```python
from build123d import *

# Parameters (mm, degrees)
SKETCH1_W           = 25.4
SKETCH1_H           = 25.4
BOSS_EXTRUDE1_DEPTH = 19.05
BOSS_EXTRUDE2_DEPTH = 25.4


with BuildPart() as part:
    # Sketch1 → Boss-Extrude1 (new body)
    with BuildSketch(Plane(origin=(0, 0, 0), x_dir=(1, 0, 0), z_dir=(0, 1, 0))):
        with Locations((12.7, 12.7)):
            Rectangle(SKETCH1_W, SKETCH1_H)
    extrude(amount=BOSS_EXTRUDE1_DEPTH)

    # Sketch3 → Boss-Extrude2 (add)
    with BuildSketch(Plane(origin=(0, 19.05, 0), x_dir=(1, 0, 0), z_dir=(0, 1, 0))):
        with BuildLine():
            Line((0, 0), (0, 9.1694))
            ThreePointArc((0, 9.1694), (6.483744919, 6.483744919), (9.1694, 0))
            Line((9.1694, 0), (0, 0))
        make_face()
    extrude(amount=BOSS_EXTRUDE2_DEPTH)


solid = part.part
```
Check sheet for the modelled part. Datum: model origin and axes. Units: mm. A direction names the side the tool comes from. Round coordinates to 2 decimals unless told otherwise and drop trailing zeros. Order: outer loops, then holes, each group sorted by start corner. A loop starts at its lowest first (then second) coordinate and runs counter-clockwise, first axis right, second up.
1) Section check D-D (x = 19.75). Record the boundary of the cut face in (y, z), and give its area (3 significant figures).
2) Section check B-B (x = 6.5). Record the boundary of the cut face in (y, z), and give its area (3 significant figures).
3) Section check A-A (z = -10). Record the boundary of the cut face in (x, y).
4) Scan lines: line 1 (Y direction, x = 19, z = -15.5); line 2 (X direction, y = 33, z = -2.5); line 3 (Z direction, x = 6.75, y = 23). Record each from-to range of solid material in increasing order.
5) Go/stop test with a flat-tipped pin: pin 1 Ø8 at (x, z) = (16.5, -11) entering from +Y. Record where the tip stops, or that it passes through.
6) Tool access check on faces 1 (the flat face through (13, 19.05, -13)), 2 (the flat face through (25.4, 9, -13)). Record the directions out of +Z, -Z, +X, -X, +Y, -Y that give a thin tool (end or side, any length) a straight path to the whole face; none if there is none.
7) Section check C-C (y = 29). Record the boundary of the cut face in (x, z).
Result:
1. outline: (0, -25.4) - (19.05, -25.4) - (19.05, 0) - (0, 0) - close
1. area: 484 mm2
2. outline: (0, -25.4) - (19.05, -25.4) - (19.05, -6.47) - (44.45, -6.47) - (44.45, 0) - (0, 0) - close
2. area: 648 mm2
3. outline: (0, 0) - (25.4, 0) - (25.4, 19.05) - (0, 19.05) - close
4. line 1: y = 0 to 19.05
4. line 2: x = 0 to 8.82
4. line 3: z = -6.21 to 0
5. pin 1: stops at y = 19.05
6. face 1: -Z, +X, +Y
6. face 2: +Z, -Z, +X, +Y, -Y
7. outline: (0, -9.17) arc R9.17 ccw to (9.17, 0) - (0, 0) - close
